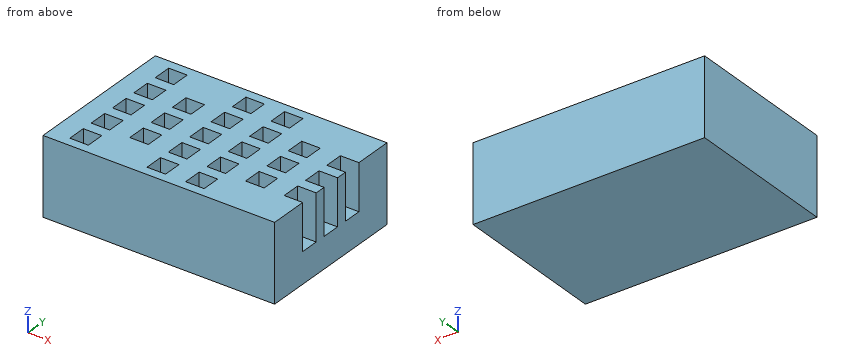
```python
from build123d import *

# Parameters (mm, degrees)
SKETCH_1_W          = 15
SKETCH_1_H          = 10
EXTRUDE_1_DEPTH     = 5
SKETCH_2_W          = 1.2
SKETCH_2_H          = 1.2
CUT_EXTRUDE_1_DEPTH = 3


with BuildPart() as part:
    # 草图1 → 凸台-拉伸1 (new body)
    with BuildSketch(Plane.XY):
        with Locations((7.5, -5)):
            Rectangle(SKETCH_1_W, SKETCH_1_H)
    extrude(amount=EXTRUDE_1_DEPTH)

    # 草图2 → 切除-拉伸1 (cut)
    with BuildSketch(Plane.XY.offset(5)):
        with Locations((1.9, -1.2)):
            Rectangle(SKETCH_2_W, SKETCH_2_H)
        with Locations((1.9, -3.1)):
            Rectangle(SKETCH_2_W, SKETCH_2_H)
        with Locations((1.9, -5)):
            Rectangle(SKETCH_2_W, SKETCH_2_H)
        with Locations((1.9, -6.9)):
            Rectangle(SKETCH_2_W, SKETCH_2_H)
        with Locations((1.9, -8.8)):
            Rectangle(SKETCH_2_W, SKETCH_2_H)
        with Locations((4.4, -3.1)):
            Rectangle(SKETCH_2_W, SKETCH_2_H)
        with Locations((6.9, -3.1)):
            Rectangle(SKETCH_2_W, SKETCH_2_H)
        with Locations((11.9, -3.1)):
            Rectangle(SKETCH_2_W, SKETCH_2_H)
        with Locations((9.4, -3.1)):
            Rectangle(SKETCH_2_W, SKETCH_2_H)
        with Locations((14.4, -3.1)):
            Rectangle(SKETCH_2_W, SKETCH_2_H)
        with Locations((4.4, -5)):
            Rectangle(SKETCH_2_W, SKETCH_2_H)
        with Locations((6.9, -5)):
            Rectangle(SKETCH_2_W, SKETCH_2_H)
        with Locations((9.4, -5)):
            Rectangle(SKETCH_2_W, SKETCH_2_H)
        with Locations((11.9, -5)):
            Rectangle(SKETCH_2_W, SKETCH_2_H)
        with Locations((14.4, -5)):
            Rectangle(SKETCH_2_W, SKETCH_2_H)
        with Locations((4.4, -6.9)):
            Rectangle(SKETCH_2_W, SKETCH_2_H)
        with Locations((6.9, -6.9)):
            Rectangle(SKETCH_2_W, SKETCH_2_H)
        with Locations((9.4, -6.9)):
            Rectangle(SKETCH_2_W, SKETCH_2_H)
        with Locations((11.9, -6.9)):
            Rectangle(SKETCH_2_W, SKETCH_2_H)
        with Locations((14.4, -6.9)):
            Rectangle(SKETCH_2_W, SKETCH_2_H)
        with Locations((6.9, -8.8)):
            Rectangle(SKETCH_2_W, SKETCH_2_H)
        with Locations((9.4, -8.8)):
            Rectangle(SKETCH_2_W, SKETCH_2_H)
        with Locations((6.9, -1.2)):
            Rectangle(SKETCH_2_W, SKETCH_2_H)
        with Locations((9.4, -1.2)):
            Rectangle(SKETCH_2_W, SKETCH_2_H)
    extrude(amount=-CUT_EXTRUDE_1_DEPTH, mode=Mode.SUBTRACT)


solid = part.part
```
Can you work these out from the model? Positions are in its coordinate system, mm. Round coordinates to 2 decimals unless told otherwise and drop trailing zeros. Loops run counter-clockwise (first coordinate to the right, second up) from the corner with the lowest first, then second, coordinate; pieces in that order, holes last. Notation, with made-up numbers: M 54,1.5 L 98,1.5 A22 ccw 98,27.5 Z; hole C 75.25,44.25 d5. An arc over 180 degrees is marked long. Answer in a Markdown table with one row per item.
1. If we section it at D-D, the plane y = -7: Please give me the cut outline in (x, z).
Established:
| item | result |
|---|---|
| outline | M 0,0 L 15,0 L 15,2 L 13.8,2 L 13.8,5 L 12.5,5 L 12.5,2 L 11.3,2 L 11.3,5 L 10,5 L 10,2 L 8.8,2 L 8.8,5 L 7.5,5 L 7.5,2 L 6.3,2 L 6.3,5 L 5,5 L 5,2 L 3.8,2 L 3.8,5 L 2.5,5 L 2.5,2 L 1.3,2 L 1.3,5 L 0,5 Z |
2. If we section it at C-C, the plane z = 3.2: Give the number of separate pieces and of enclosed holes in the cut face, plus the area to 3 significant figures.
Established:
| item | result |
|---|---|
| separate pieces | 1 |
| enclosed holes | 21 |
| area | 115 mm² |
3. If we section it at B-B, the plane x = 6.5: Please give me the cut outline in (y, z).
Established:
| item | result |
|---|---|
| outline | M -10,0 L 0,0 L 0,5 L -0.6,5 L -0.6,2 L -1.8,2 L -1.8,5 L -2.5,5 L -2.5,2 L -3.7,2 L -3.7,5 L -4.4,5 L -4.4,2 L -5.6,2 L -5.6,5 L -6.3,5 L -6.3,2 L -7.5,2 L -7.5,5 L -8.2,5 L -8.2,2 L -9.4,2 L -9.4,5 L -10,5 Z |
4. Please list where these lines run through material, in increasing order: line 1 (X direction, y = -5.25, z = 2.85); line 2 (Y direction, x = 9, z = 2.7); line 3 (X direction, y = -8.25, z = 4.75). Write a range as from..to.
Established:
| item | result |
|---|---|
| line 1 | 0..1.3, 2.5..3.8, 5..6.3, 7.5..8.8, 10..11.3, 12.5..13.8 |
| line 2 | -10..-9.4, -8.2..-7.5, -6.3..-5.6, -4.4..-3.7, -2.5..-1.8, -0.6..0 |
| line 3 | 0..1.3, 2.5..6.3, 7.5..8.8, 10..15 |
5. I'm going to push flat-ended pins straight in: pin 1 Ø0.6 at (x, y) = (12, -5) entering from +Z; pin 2 Ø0.6 at (y, z) = (-3, 3.5) entering from +X. Where does each tip first touch, or does it pass through?
Established:
| item | result |
|---|---|
| pin 1 | z = 2 |
| pin 2 | x = 13.8 |
6. If we section it at A-A, the plane y = -8.75: Please give me the cut outline in (x, z), plus the area to 3 significant figures.
Established:
| item | result |
|---|---|
| outline | M 0,0 L 15,0 L 15,5 L 10,5 L 10,2 L 8.8,2 L 8.8,5 L 7.5,5 L 7.5,2 L 6.3,2 L 6.3,5 L 2.5,5 L 2.5,2 L 1.3,2 L 1.3,5 L 0,5 Z |
| area | 64.2 mm² |
